Check sheet for the modelled part. Datum: model origin and axes. Units: mm. Face numbers are marked on the shaded views. A direction names the side the tool comes from. Round coordinates to 2 decimals unless told otherwise and drop trailing zeros. Write each loop counter-clockwise with the first axis right and the second up, starting at its lowest first coordinate (ties: lowest second). Pieces come first, ordered by that corner, then holes. Notation, with made-up numbers: M -4,-29.75 L 19,-29.75 A24 cw 19,6.25 Z; hole C -28.5,12.25 d8. An arc over 180 degrees is marked long. Answer in a Markdown table with one row per item.
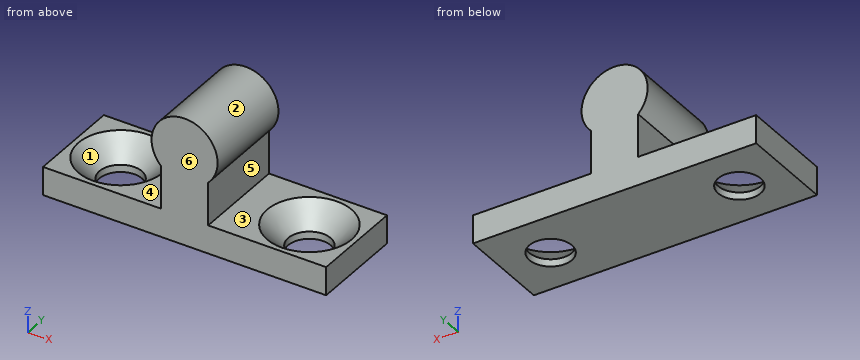
```python
from build123d import *

# Parameters (mm, degrees)
SKETCH_1_W                  = 30
SKETCH_1_H                  = 3
EXTRUDE_1_DEPTH             = 5
HOLE_WIZARD_M4_1_AT_2_COUNT = 2
HOLE_WIZARD_M4_1_AT_2_PITCH = 20


with BuildPart() as part:
    # 草图1 → 拉伸1 (new, symmetric)
    with BuildSketch(Plane(origin=(0, 0, 0), x_dir=(1, 0, 0), z_dir=(0, 1, 0))):
        with BuildLine():
            Line((2.5, -3), (-2.5, -3))
            Line((-2.5, -3), (-2.5, -7.550510257))
            ThreePointArc((-2.5, -7.550510257), (0, -13.5), (2.5, -7.550510257))
            Line((2.5, -7.550510257), (2.5, -3))
        make_face()
        with Locations((0, -1.5)):
            Rectangle(SKETCH_1_W, SKETCH_1_H)
    extrude(amount=EXTRUDE_1_DEPTH, both=True)

    # 草图2 → M4 六角凹锥坑螺钉的锥形沉头孔1 (revolve, cut)
    with BuildSketch(Plane(origin=(-10, 0, 3), x_dir=(0, -1, 0), z_dir=(1, 0, 0))):
        Polygon((0, 0), (0, 3), (2.25, 3), (2.25, 2.23), (4.48, 0), align=None)
    hole_wizard_m4_1 = revolve(axis=Axis((-10, 0, 9.35), (0, 0, -1)), mode=Mode.SUBTRACT)

    # M4 六角凹锥坑螺钉的锥形沉头孔1 at 2: M4 六角凹锥坑螺钉的锥形沉头孔1 ×2
    with Locations(*[(i * HOLE_WIZARD_M4_1_AT_2_PITCH, 0, 0) for i in range(1, HOLE_WIZARD_M4_1_AT_2_COUNT)]):
        add(hole_wizard_m4_1, mode=Mode.SUBTRACT)


solid = part.part
```
1. Access from +Z, -Z, +X, -X, +Y, -Y to the whole of each face (thin tool, end or side, straight path). Record for the marked faces 4, 5 and 6.
Found:
| item | result |
|---|---|
| face 4 | -X, +Y, -Y |
| face 5 | +X, +Y, -Y |
| face 6 | +Z, -Z, +X, -X, -Y |
2. Draft check along X on the marked faces 1, 2 and 3. Enter one of: +X half, -X half, draft (parallel to the pull), parting line (faces both ways), or undercut.
Found:
| item | result |
|---|---|
| face 1 | undercut |
| face 2 | parting line |
| face 3 | draft |
3. Section check B-B, the plane z = 1.25. Record the cut outline in (x, y), and give its area (3 significant figures).
Found:
| item | result |
|---|---|
| outline | M -15,-5 L 15,-5 L 15,5 L -15,5 Z; hole C -10,0 d5.46; hole C 10,0 d5.46 |
| area | 253 mm2 |
4. Section check C-C, the plane z = 6.75. Record the cut outline in (x, y).
Found:
| item | result |
|---|---|
| outline | M -2.5,-5 L 2.5,-5 L 2.5,5 L -2.5,5 Z |
5. Section check A-A, the plane x = -10. Record the cut outline in (y, z), and give its area (3 significant figures).
Found:
| item | result |
|---|---|
| outline | M -5,0 L -2.25,0 L -2.25,0.77 L -4.48,3 L -5,3 Z; M 2.25,0 L 5,0 L 5,3 L 4.48,3 L 2.25,0.77 Z |
| area | 11.5 mm2 |
6. Section check D-D, the plane y = 0.75. Count the separate pieces of the cut face and the enclosed holes in it, and give its area (3 significant figures).
Found:
| item | result |
|---|---|
| separate pieces | 3 |
| enclosed holes | 0 |
| area | 112 mm2 |
7. Scan lines: L1, parallel to X at y = 0, z = 0.5; L2, parallel to Y at x = 10, z = 0.55; L3, parallel to X at y = 2.25, z = 3.5. Record each from-to range of solid material in increasing order.
Found:
| item | result |
|---|---|
| L1 | x = -15 to -12.25, -7.75 to 7.75, 12.25 to 15 |
| L2 | y = -5 to -2.25, 2.25 to 5 |
| L3 | x = -2.5 to 2.5 |
8. Go/stop test with flat-tipped pins: pin 1 (5 mm diameter, centred on x = 6.5, y = 0, fed in from +Z); pin 2 (2.5 mm diameter, centred on y = -2, z = 5.5, fed in from +X); pin 3 (2.5 mm diameter, centred on y = -2, z = 4.5, fed in from -X). Record where each tip stops, or that it passes through.
Found:
| item | result |
|---|---|
| pin 1 | stops at z = 3 |
| pin 2 | stops at x = 2.5 |
| pin 3 | stops at x = -2.5 |
